Source: CAD feature listing. Evaluate the final solid. Frame: model axes, mm. Round coordinates to 2 decimals unless told otherwise and drop trailing zeros. Loops run counter-clockwise (first coordinate to the right, second up) from the corner with the lowest first, then second, coordinate; pieces in that order, holes last. Notation, with made-up numbers: M 38.25,-33 L 48.25,-33 A15 ccw 48.25,-27 Z; hole C 70,-5.75 d11. An arc over 180 degrees is marked long. One line per item, written item: value.
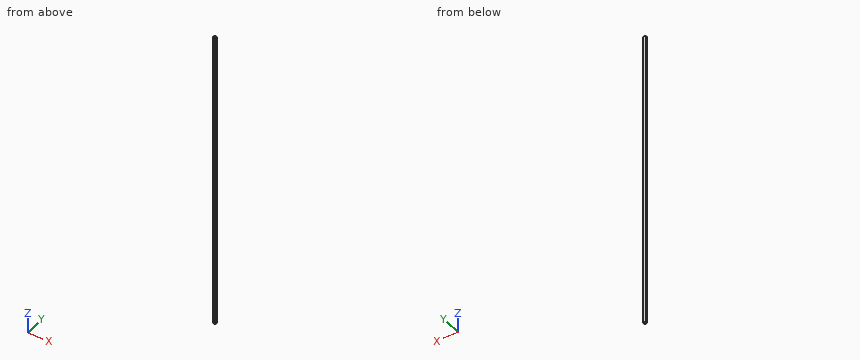
from build123d import *

# Parameters (mm, degrees)
EXTRUDE_1_DEPTH = 1000


with BuildPart() as part:
    # Эскиз1 → Бобышка-Вытянуть1 (new body)
    with BuildSketch(Plane.XY):
        with BuildLine():
            Line((0, 0), (-5.2, 3.0022214))
            Line((-5.2, 3.0022214), (-4.7, 3.868246804))
            Line((-4.7, 3.868246804), (-4.7, 7.074937186))
            Line((-4.7, 7.074937186), (-5.204805472, 7.074937186))
            ThreePointArc((-5.204805472, 7.074937186), (0, 9.3), (5.204805472, 7.074937186))
            Line((5.204805472, 7.074937186), (4.7, 7.074937186))
            Line((4.7, 7.074937186), (4.7, 3.868246804))
            Line((4.7, 3.868246804), (5.2, 3.0022214))
            Line((5.2, 3.0022214), (0, 0))
        make_face()
        with BuildLine():
            Line((0, 1.154700538), (-3.7, 3.290896534))
            Line((-3.7, 3.290896534), (-3.7, 7.074937186))
            ThreePointArc((-3.7, 7.074937186), (0, 8.3), (3.7, 7.074937186))
            Line((3.7, 7.074937186), (3.7, 3.290896534))
            Line((3.7, 3.290896534), (0, 1.154700538))
        make_face(mode=Mode.SUBTRACT)
    extrude(amount=EXTRUDE_1_DEPTH)


solid = part.part
1. Ray query, line 1 (X direction, y = 6.75, z = 253.5); line 2 (Y direction, x = -1, z = 852); line 3 (Y direction, x = 3.25, z = 208). Return the intervals inside material, ascending. Write a range as [from, to].
Report:
line 1: x = [-4.7, -3.7], [3.7, 4.7]
line 2: y = [0.58, 1.73], [8.22, 9.23]
line 3: y = [1.88, 3.03], [7.38, 8.52]
2. Pin query (flat end, axial travel): pin 1 (6 mm diameter, centred on x = -2, z = 712, fed in from +Y); pin 2 (3.5 mm diameter, centred on y = 5.5, z = 617.5, fed in from -X); pin 3 (1.9 mm diameter, centred on y = 6, z = 721.5, fed in from -X); pin 4 (1.5 mm diameter, centred on y = 2.5, z = 273, fed in from +X). Return the tip coordinate at first contact, or that it passes through.
Report:
pin 1: stops at y = 9.3
pin 2: stops at x = -5.2
pin 3: stops at x = -4.7
pin 4: stops at x = 5.2
3. Section query C-C (x = 2). Return the cut outline in (y, z), and give its area (3 significant figures).
Report:
outline: M 1.15,0 L 2.31,0 L 2.31,1000 L 1.15,1000 Z; M 7.97,0 L 9.02,0 L 9.02,1000 L 7.97,1000 Z
area: 2,200 mm2
4. Section query A-A (y = 5.5). Return the cut outline in (x, z), and give its area (3 significant figures).
Report:
outline: M -4.7,0 L -3.7,0 L -3.7,1000 L -4.7,1000 Z; M 3.7,0 L 4.7,0 L 4.7,1000 L 3.7,1000 Z
area: 2,000 mm2
5. Section query B-B (z = 351.5). Return the cut outline in (x, y), and give its area (3 significant figures).
Report:
outline: M -5.2,3 L 0,0 L 5.2,3 L 4.7,3.87 L 4.7,7.07 L 5.2,7.07 A7.2 ccw -5.2,7.07 L -4.7,7.07 L -4.7,3.87 Z; hole M -3.7,3.29 L 0,1.15 L 3.7,3.29 L 3.7,7.07 A6.2 ccw -3.7,7.07 Z
area: 28.2 mm2
